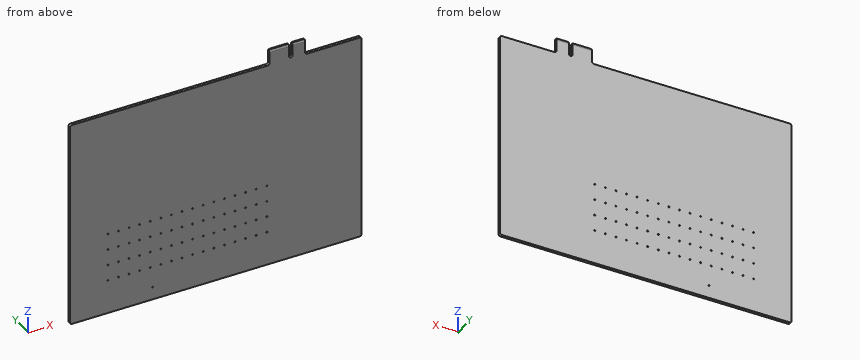
from build123d import *

# Parameters (mm, degrees)
SKETCH1_W                    = 165
SKETCH1_H                    = 129
BOSS_EXTRUDE1_DEPTH          = 1.6
SKETCH2_W                    = 112.85
SKETCH2_H                    = 9
CUT_EXTRUDE1_DEPTH           = 224.491744814
SKETCH3_W                    = 31.85
SKETCH3_H                    = 9
CUT_EXTRUDE2_DEPTH           = 224.491744814
SKETCH4_W                    = 1.9
SKETCH4_H                    = 8.41
CUT_EXTRUDE3_DEPTH           = 224.491744814
FILLET1_R                    = 1
FILLET2_R                    = 0.95
CHAMFER1_SIZE                = 0.5
F_0_65_0_65_DIAMETER_HOLE1_D = 0.65
LPATTERN1_COUNT              = 16
LPATTERN1_PITCH              = 6
LPATTERN1_COUNT_DIR2         = 4
LPATTERN1_PITCH_DIR2         = 9.302
F_0_65_0_65_DIAMETER_HOLE2_D = 0.65
CUT_EXTRUDE4_DEPTH           = 216.751152952


with BuildPart() as part:
    # Sketch1 → Boss-Extrude1 (new body)
    with BuildSketch(Plane(origin=(0, 0, 0), x_dir=(1, 0, 0), z_dir=(0, 1, 0))):
        with Locations((92.5, 74.5)):
            Rectangle(SKETCH1_W, SKETCH1_H)
    extrude(amount=BOSS_EXTRUDE1_DEPTH)

    # Sketch2 → Cut-Extrude1 (cut, through all)
    with BuildSketch(Plane(origin=(0, 1.6, 0), x_dir=(1, 0, 0), z_dir=(0, 1, 0))):
        with Locations((66.425, 14.5)):
            Rectangle(SKETCH2_W, SKETCH2_H)
    extrude(amount=-CUT_EXTRUDE1_DEPTH, mode=Mode.SUBTRACT)

    # Sketch3 → Cut-Extrude2 (cut, through all)
    with BuildSketch(Plane(origin=(0, 1.6, 0), x_dir=(1, 0, 0), z_dir=(0, 1, 0))):
        with Locations((159.075, 14.5)):
            Rectangle(SKETCH3_W, SKETCH3_H)
    extrude(amount=-CUT_EXTRUDE2_DEPTH, mode=Mode.SUBTRACT)

    # Sketch4 → Cut-Extrude3 (cut, through all)
    with BuildSketch(Plane(origin=(0, 1.6, 0), x_dir=(1, 0, 0), z_dir=(0, 1, 0))):
        with Locations((135, 14.205)):
            Rectangle(SKETCH4_W, SKETCH4_H)
    extrude(amount=-CUT_EXTRUDE3_DEPTH, mode=Mode.SUBTRACT)

    # Fillet1
    fillet1_edges = [part.edges().sort_by_distance(p)[0] for p in [
        (10, 0.8, -19),
        (122.85, 0.8, -19),
        (175, 0.8, -19),
        (143.15, 0.8, -19),
        (10, 0.8, -139),
        (175, 0.8, -139),
    ]]
    fillet(fillet1_edges, radius=FILLET1_R)

    # Fillet2
    fillet2_edges = [part.edges().sort_by_distance(p)[0] for p in [
        (135.95, 0.8, -18.41),
        (134.05, 0.8, -18.41),
    ]]
    fillet(fillet2_edges, radius=FILLET2_R - 0.0001)  # a hair under: the kernel refuses the full size

    # Chamfer1
    chamfer1_edges = [part.edges().sort_by_distance(p)[0] for p in [
        (122.85, 0.8, -10),
        (143.15, 0.8, -10),
        (135.95, 0.8, -10),
        (134.05, 0.8, -10),
    ]]
    chamfer(chamfer1_edges, length=CHAMFER1_SIZE)

    # Ø0.65 (0.65) Diameter Hole1 (through all)
    with Locations(Plane(origin=(0, 1.6, 0), x_dir=(1, 0, 0), z_dir=(0, 1, 0))):
        with Locations((31.402, 91.42)):
            f_0_65_0_65_diameter_hole1 = Hole(F_0_65_0_65_DIAMETER_HOLE1_D / 2)

    # LPattern1: 0.65 _0.65_ Diameter Hole1 16 × 4
    with Locations(*[(i * LPATTERN1_PITCH, 0, -j * LPATTERN1_PITCH_DIR2) for i in range(LPATTERN1_COUNT) for j in range(LPATTERN1_COUNT_DIR2) if (i, j) != (0, 0)]):
        add(f_0_65_0_65_diameter_hole1, mode=Mode.SUBTRACT)

    # Ø0.65 (0.65) Diameter Hole2 (through all)
    with Locations(Plane(origin=(0, 1.6, 0), x_dir=(1, 0, 0), z_dir=(0, 1, 0))):
        with Locations((56.694, 131.618)):
            Hole(F_0_65_0_65_DIAMETER_HOLE2_D / 2)

    # Sketch11 → Cut-Extrude4 (cut, through all)
    with BuildSketch(Plane(origin=(175, 0, 0), x_dir=(0, 0, -1), z_dir=(1, 0, 0))):
        Polygon((11.3, 1.6), (10, 1.126838695), (10, 1.6), align=None)
        Polygon((11.3, 0), (10, 0), (10, 0.473161305), align=None)
    extrude(amount=-CUT_EXTRUDE4_DEPTH, mode=Mode.SUBTRACT)


solid = part.part
Geometry: final body of the model. Coordinates: model frame, mm. Coordinates: 2 decimals unless noted, no trailing zeros. Loops run counter-clockwise (first coordinate to the right, second up) from the corner with the lowest first, then second, coordinate; pieces in that order, holes last. Notation, with made-up numbers: M 40,-26 L 98,-26 A36 cw 98,8 Z; hole C 35.5,-8 d7. An arc over 180 degrees is marked long. One line per item, written item: value. Start each with the question number.
1) Pin query (flat end, axial travel): P1, Ø0.5, axis at y = 0.5, z = -12.5, coming from the +X side; P2, Ø6, axis at x = 115, z = -109.5, coming from the -Y side; P3, Ø0.5, axis at x = 50.5, y = 0.5, coming from the +Z side; P4, Ø0.8, axis at y = 1, z = -13, coming from the -X side. Return the tip coordinate at first contact, or that it passes through.
2) Cut plane A-A (x = 21). Return loops of the section in (y, z), then the cut area to 3 significant figures.
3) Material intervals for L1, parallel to Z at x = 31.5, y = 1.3; L2, parallel to Z at x = 74.5, y = 1.1, sorted ascending. Write a range as from..to.
Evaluation:
1. P1: x = 143.15
1. P2: y = 0
1. P3: z = -19
1. P4: x = 122.85
2. outline: M 0,-139 L 1.6,-139 L 1.6,-19 L 0,-19 Z
2. area: 192 mm^2
3. L1: -139..-119.64, -119.02..-110.33, -109.71..-101.03, -100.41..-91.73, -91.11..-19
3. L2: -139..-19
